Autodesk Inventor part; units mm, degrees
ref_plane "YZ Plane" through (0, 0, 0) normal (1, 0, 0) x (0, 1, 0)
ref_plane "XZ Plane" through (0, 0, 0) normal (0, 1, 0) x (-1, 0, 0)
ref_plane "XY Plane" through (0, 0, 0) normal (0, 0, 1) x (1, 0, 0)
sketch "草圖1" plane through (0, 0, 0) normal (0, 1, 0) x (-1, 0, 0)
  line L0 (2.5, 12.5) -> (-2.5, 12.5)
  line L1 (-2.5, 12.5) -> (-2.5, -12.5)
  line L2 (-2.5, -12.5) -> (2.5, -12.5)
  line L3 (2.5, -12.5) -> (2.5, 12.5)
  circle A0 centre (0, 10) radius 1.7
  circle A1 centre (0, 5) radius 1.7
  circle A2 centre (0, 0) radius 1.7
  circle A3 centre (0, -5) radius 1.7
  circle A4 centre (0, -10) radius 1.7
  point P0 (0, 0)
  point P1 (2.5, 0)
  point P2 (0, 12.5)
  dimension "d0" = 5
  dimension "d1" = 25
  dimension "d2" = 3.4
  dimension "d3" = 2.5
  dimension "d4" = 2.5
  dimension "d7" = 5
sketch "草圖2" plane through (0, 0, 0) normal (1, 0, 0) x (0, 1, 0)
  line L0 (0, -12.5) -> (0, 12.5)
  circle A0 centre (0, 0) radius 7.5
  line L1 (0, 12.5) -> (10, 12.5)
  line L2 (10, 12.5) -> (10, -12.5)
  line L3 (10, -12.5) -> (0, -12.5)
  point P0 (0, 10)
  point P1 (0, 5)
  point P2 (0, -5)
  point P3 (0, -10)
  point P4 (0, 7.5)
  point P5 (0, -7.5)
  dimension "d12" = 15
  dimension "d13" = 10
extrude "擠出1" add sketch "草圖2" along normal mid plane 5 contours L0 A0 L1 L2 L3
extrude "擠出2" cut sketch "草圖1" along normal blind 1.5 contours A0 | A4
properties part number "110033226_ipt_09_窗戶圓拱"
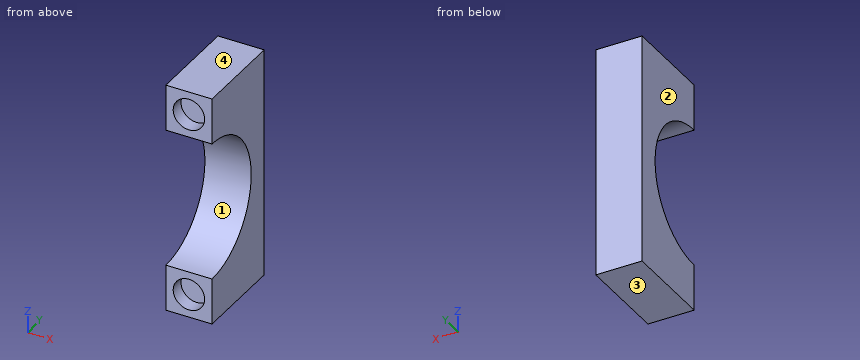
For this review, take the finished solid that the model builds, in its own axes (mm). Face numbers are marked on the shaded views. Give positions to 0.01 mm unless a question says otherwise; leave off trailing zeros. Order: outer loops, then holes, each group sorted by start corner. A loop starts at its lowest first (then second) coordinate and runs counter-clockwise, first axis right, second up. Notation, with made-up numbers: (41, 20.25) - (75, 20.25) arc R16 cw to (75, 30.25) - close; hole circle Ø1 at (36.5, 89.25). An arc over 180 degrees is marked (long way). Answer as a JSON object with one key per item and string values. Group by question number.
Item 1: Wall thickness on line 1 along Z through (x, y) = (0, 1.1); line 2 along Z through (x, y) = (-1.1, 1); line 3 along Y through (x, z) = (-1.15, 10.75): over which ranges is each line inside the solid? List them lowest first.
Item 2: Take a section at B-B on z = 10. Give the boundary of the cut face in (x, y), and give its area (3 significant figures).
Item 3: Draft analysis for pull direction Z (two halves, no side actions). For the marked faces 1, 2, 3 and 4, state which applies: pulls with the +Z half, pulls with the -Z half, needs draft (parallel to the pull), parting line crosses it, or undercut.
Item 4: Clearance check with a flat-ended pin moving along its axis: pin 1 Ø2.5 at (x, z) = (0, 10) entering from -Y. State where the tip first meets the part, or that it passes through.
Item 5: Take a section at D-D on y = 2.5. Give the boundary of the cut face in (x, z), and give its area (3 significant figures).
Item 6: Take a section at C-C on x = 0. Give the boundary of the cut face in (y, z), and give its area (3 significant figures).
Item 7: Take a section at A-A on y = 4.5. Give the boundary of the cut face in (x, z), and give its area (3 significant figures).
Reported:
{
 "1": {"line 1": "-12.5 to -11.7, -8.3 to -7.42, 7.42 to 8.3, 11.7 to 12.5", "line 2": "-12.5 to -11.3, -8.7 to -7.43, 7.43 to 8.7, 11.3 to 12.5", "line 3": "1.5 to 10"},
 "2": {"outline": "(-2.5, 0) - (-1.7, 0) - (-1.7, 1.5) - (1.7, 1.5) - (1.7, 0) - (2.5, 0) - (2.5, 10) - (-2.5, 10) - close", "area": "44.9 mm^2"},
 "3": {"face 1": "undercut", "face 2": "needs draft", "face 3": "pulls with the -Z half", "face 4": "pulls with the +Z half"},
 "4": {"pin 1": "y = 1.5"},
 "5": {"outline": "(-2.5, -12.5) - (2.5, -12.5) - (2.5, -7.07) - (-2.5, -7.07) - close; (-2.5, 7.07) - (2.5, 7.07) - (2.5, 12.5) - (-2.5, 12.5) - close", "area": "54.3 mm^2"},
 "6": {"outline": "(0, -12.5) - (10, -12.5) - (10, 12.5) - (0, 12.5) - (0, 11.7) - (1.5, 11.7) - (1.5, 8.3) - (0, 8.3) - (0, 7.5) arc R7.5 cw to (0, -7.5) - (0, -8.3) - (1.5, -8.3) - (1.5, -11.7) - (0, -11.7) - close", "area": "151 mm^2"},
 "7": {"outline": "(-2.5, -12.5) - (2.5, -12.5) - (2.5, -6) - (-2.5, -6) - close; (-2.5, 6) - (2.5, 6) - (2.5, 12.5) - (-2.5, 12.5) - close", "area": "65.0 mm^2"}
}
